Autodesk Fusion 360 part; units mm, degrees
sketch "スケッチ1" plane through (0, 0, 0) normal (0, 0, 1) x (1, 0, 0)
  circle A0 centre (0, 0) radius 3.45
  line L0 (3.1177, 0) -> (1.5588, 2.7)
  line L1 (1.5588, 2.7) -> (-1.5588, 2.7)
  line L2 (-1.5588, 2.7) -> (-3.1177, 0)
  line L3 (-3.1177, 0) -> (-1.5588, -2.7)
  line L4 (-1.5588, -2.7) -> (1.5588, -2.7)
  line L5 (1.5588, -2.7) -> (3.1177, 0)
  dimension "d1" = 6.9
  dimension "d2" = 5.4
extrude "押し出し1" add sketch "スケッチ1" along normal blind 8
Can you work these out from the model? Positions are in its coordinate system, mm. A direction names the side the tool comes from. Coordinates: 2 decimals unless noted, no trailing zeros. Write each loop counter-clockwise with the first axis right and the second up, starting at its lowest first coordinate (ties: lowest second). Pieces come first, ordered by that corner, then holes. Notation, with made-up numbers: M -38,72.5 L 5,72.5 A6 ccw 5,77.5 Z; hole C -39.5,-20.75 d9. An arc over 180 degrees is marked long. Use one line per item in the form item = value.
Q1. We'd pull the mould along X, two halves only. Please class faces 3 (the flat face through (-3, 1, 8)), 4 (the cylindrical face through (-0.45, -3.42, 3.94)), 5 (the flat face through (2.327, -1.369, 3.944)), 6 (the flat face through (0, 2.7, 4)): +X half, -X half, draft (parallel to the pull), parting line (faces both ways), or undercut.
Model answer:
face_3 = draft
face_4 = parting line
face_5 = undercut
face_6 = undercut
Q2. For faces 1 (the flat face through (2.35, 1.33, 3.94)), 2 (the flat face through (-3, 1, 0)), which set-ups out of +Z, -Z, +X, -X, +Y, -Y let a thin tool reach every point of the face, with its end or its side?
Model answer:
face_1 = +Z, -Z
face_2 = -Z, +X, -X, +Y, -Y
Q3. If we section it at A-A (z = 4.75): Write out the boundary of the cut face in (x, y), then the cut area to 3 significant figures.
Model answer:
outline = C 0,0 d6.9; hole M -3.12,0 L -1.56,-2.7 L 1.56,-2.7 L 3.12,0 L 1.56,2.7 L -1.56,2.7 Z
area = 12.1 mm^2
Q4. If we section it at B-B (x = 3): Write out the boundary of the cut face in (y, z).
Model answer:
outline = M -1.7,0 L -0.2,0 L -0.2,8 L -1.7,8 Z; M 0.2,0 L 1.7,0 L 1.7,8 L 0.2,8 Z
Q5. If we section it at C-C (y = -1): Write out the boundary of the cut face in (x, z), then the cut area to 3 significant figures.
Model answer:
outline = M -3.3,0 L -2.54,0 L -2.54,8 L -3.3,8 Z; M 2.54,0 L 3.3,0 L 3.3,8 L 2.54,8 Z
area = 12.2 mm^2
Q6. For P1, Ø2.5, axis at x = 0.5, z = 3, coming from the +Y side; P2, Ø1.5, axis at x = 2.5, z = 2.5, coming from the +Y side; P3, Ø2, axis at y = -1.5, z = 2, coming from the -X side; P4, Ø3, axis at y = -2, z = 1.5, coming from the +X side, each with a flat end and sliding along its axis, tell me the tip position at first contact or that it passes through.
Model answer:
P1 = 3.45
P2 = 2.97
P3 = -3.41
P4 = 3.41
Q7. I need wall thicknesses on line 1 along X through (y, z) = (-0.25, 3); line 2 along X through (y, z) = (2.5, 3.5); line 3 along Y through (x, z) = (1, 0.75). Which ranges of each line are inside material? Lowest first, please. Write a range as from..to.
Model answer:
line_1 = -3.44..-2.97, 2.97..3.44
line_2 = -2.38..-1.67, 1.67..2.38
line_3 = -3.3..-2.7, 2.7..3.3
